from build123d import *

# Parameters (mm, degrees)
F1_DEPTH  = 12.7
F2_W      = 9.525
F2_H      = 12.7
F2_R      = 2.54
F2_W_2    = 19.05
F3_DEPTH  = 6.35
F4_DEPTH  = 25.4
F6_DEPTH  = 12.7
F7_DEPTH  = 12.7
F8_R      = 3.8109417559
F8_R_2    = 2.54
F9_DEPTH  = 25.4
F10_R     = 3.81
F10_R_2   = 2.54
F11_DEPTH = 25.4


with BuildPart() as f1:
    # F0 (on Top) → F1 (new body)
    with BuildSketch(Plane.XY):
        Polygon((63.5, 19.05), (48.5505208253, 19.05), (31.75, 0), (-63.5, 0), (-63.5, -19.05), (63.5, -19.05), align=None)
    extrude(amount=F1_DEPTH)

    # F2 (on face) → F3 (join)
    with BuildSketch(Plane(origin=(-63.5, 0, 0), x_dir=(0, -1, 0), z_dir=(-1, 0, 0))):
        with Locations((-4.7625, 6.35)):
            Rectangle(F2_W, F2_H)
        with Locations((-5.3587416187, 5.8867353946)):
            Circle(F2_R, mode=Mode.SUBTRACT)
        with Locations((9.525, 6.35)):
            Rectangle(F2_W_2, F2_H)
        with Locations((23.8125, 6.35)):
            Rectangle(F2_W, F2_H)
        with Locations((24.0348111838, 5.8867353946)):
            Circle(F2_R, mode=Mode.SUBTRACT)
    extrude(amount=F3_DEPTH)

    # F2 (on face) → F4 (cut)
    with BuildSketch(Plane(origin=(-63.5, 0, 0), x_dir=(0, -1, 0), z_dir=(-1, 0, 0))):
        with Locations((24.0348111838, 5.8867353946)):
            Circle(F2_R)
    extrude(amount=F4_DEPTH, mode=Mode.SUBTRACT)

    # F5 (on face) → F6 (join)
    with BuildSketch(Plane.XY.offset(12.7)):
        Polygon((-55.0928376615, 0), (-63.5, 9.525), (-63.5, 0), align=None)
    extrude(amount=-F6_DEPTH)

    # F5 (on face) → F7 (join)
    with BuildSketch(Plane.XY.offset(12.7)):
        Polygon((-63.5, -19.05), (-63.5, -28.575), (-55.1101081073, -19.05), align=None)
    extrude(amount=-F7_DEPTH)

    # F8 (on face) → F9 (cut)
    with BuildSketch(Plane(origin=(-63.5, 0, 0), x_dir=(0, -1, 0), z_dir=(-1, 0, 0))):
        with Locations((-5.3587416187, 5.8867353946)):
            Circle(F8_R)
        with Locations((-5.3587416187, 5.8867353946)):
            Circle(F8_R_2, mode=Mode.SUBTRACT)
        with Locations((-5.3587416187, 5.8867353946)):
            Circle(F8_R_2)
    extrude(amount=-F9_DEPTH, mode=Mode.SUBTRACT)

    # F10 (on face) → F11 (cut)
    with BuildSketch(Plane(origin=(-63.5, 0, 0), x_dir=(0, -1, 0), z_dir=(-1, 0, 0))):
        with Locations((24.0348111838, 5.8867353946)):
            Circle(F10_R)
        with Locations((24.0348111838, 5.8867353946)):
            Circle(F10_R_2, mode=Mode.SUBTRACT)
        with Locations((24.0348111838, 5.8867353946)):
            Circle(F10_R_2)
    extrude(amount=-F11_DEPTH, mode=Mode.SUBTRACT)


solid = f1.part
CAD build for the part. Positions are in the model's coordinates, mm. A direction names the side the tool comes from. Round coordinates to 2 decimals unless told otherwise and drop trailing zeros. Write each loop counter-clockwise with the first axis right and the second up, starting at its lowest first coordinate (ties: lowest second). Pieces come first, ordered by that corner, then holes. Notation, with made-up numbers: (51, -10) -> (67, -10) arc R11 cw to (67, -6) -> close; hole circle Ø4 at (-27.75, 11). An arc over 180 degrees is marked (long way). Answer as a JSON object with one key per item and string values.
(1) Band-saw the part on C-C, the plane x = -33.5. List the corners of the cut face in (y, z).
Reported:
{"outline": "(-19.05, 0) -> (0, 0) -> (0, 12.7) -> (-19.05, 12.7) -> close"}
(2) Two-plate mould, pull along Z, no slides. Class faces 1 (the face through (-60.811, 1.724, 7.031)), 2 (the face through (-4, -4, 0)), 3 (the face through (-63.5, -25, 3)), 4 (the face through (3, -19.05, 6)): +Z half, -Z half, draft (parallel to the pull), parting line (faces both ways), or undercut.
Reported:
{"face 1": "undercut", "face 2": "-Z half", "face 3": "undercut", "face 4": "draft"}
(3) Pin check, flat tips, straight feed: P1, Ø5, axis at x = -66.5, z = 9, coming from the +Y side (3 decimals); P2, Ø3, axis at y = -24.03, z = 5.89, coming from the +X side; P3, Ø5, axis at x = 23.5, z = 3, coming from the +Y side; P4, Ø2.5, axis at y = -23.5, z = 7.5, coming from the +X side. Stop position of each tip, or through.
Reported:
{"P1": "stops at y = 9.525", "P2": "passes through", "P3": "stops at y = 0", "P4": "stops at x = -63.5"}
(4) Probe probe 1 along Y at (x, z) = (27, 12); probe 2 along X at (y, z) = (8.5, 9.5); probe 3 along X at (y, z) = (6, 10.25). List the from-to ranges inside material, lowest first. Write a range as [from, to].
Reported:
{"probe 1": "y = [-19.05, 0]", "probe 2": "x = [-69.85, -62.6], [39.25, 63.5]", "probe 3": "x = [-69.85, -60.39], [37.04, 63.5]"}
(5) Band-saw the part on B-B, the plane y = -23. List the corners of the cut face in (x, z).
Reported:
{"outline": "(-69.85, 0) -> (-58.59, 0) -> (-58.59, 2.22) -> (-63.5, 2.22) -> (-63.5, 3.57) -> (-69.85, 3.57) -> close; (-69.85, 8.21) -> (-63.5, 8.21) -> (-63.5, 9.55) -> (-58.59, 9.55) -> (-58.59, 12.7) -> (-69.85, 12.7) -> close"}
(6) Which spindle directions (+Z, -Z, +X, -X, +Y, -Y) get a long thin tool onto all of the face, cutting with end or side? Do faces 5 (the face through (-60.64, -20.23, 6.05)), 6 (the face through (-63.5, 5, 3)), 7 (the face through (-11, 0, 6)). Say none if no direction does.
Reported:
{"face 5": "+X", "face 6": "none", "face 7": "+Z, -Z, +Y"}
(7) Band-saw the part on A-A, the plane y = 6.5. List the corners of the cut face in (x, z), then the cut area to 3 significant figures.
Reported:
{"outline": "(-69.85, 0) -> (-60.83, 0) -> (-60.83, 2.25) -> (-63.5, 2.25) -> (-63.5, 3.62) -> (-69.85, 3.62) -> close; (-69.85, 8.16) -> (-63.5, 8.16) -> (-63.5, 9.52) -> (-60.83, 9.52) -> (-60.83, 12.7) -> (-69.85, 12.7) -> close; (37.48, 0) -> (63.5, 0) -> (63.5, 12.7) -> (37.48, 12.7) -> close", "area": "397 mm^2"}
